CAD build for the part. Positions are in the model's coordinates, mm. Face numbers are marked on the shaded views. A direction names the side the tool comes from. Give positions to 0.01 mm unless a question says otherwise; leave off trailing zeros. Loops run counter-clockwise (first coordinate to the right, second up) from the corner with the lowest first, then second, coordinate; pieces in that order, holes last. Notation, with made-up numbers: M -12,28 L -8,28 A30 ccw -8,61 Z; hole C 43,87.25 d9. An arc over 180 degrees is marked long. One line per question, with ' | ' between items.
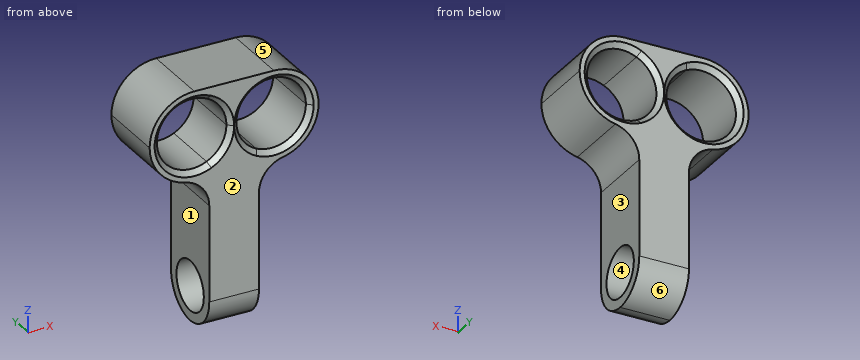
```python
from build123d import *

# Parameters (mm, degrees)
F0_W     = 5
F0_H     = 16
F1_DEPTH = 7
F3_D     = 5
F4_R     = 4.49999
F5_R     = 3.49999
F6_R     = 3
F7_SIZE  = 0.49999


# Not quite as in the source:
# - a fillet or chamfer is up to 0.001 mm smaller than in the source, because OpenCascade refuses the exact size


with BuildPart() as f1:
    # F0 (on Front) → F1 (new body)
    with BuildSketch(Plane.XZ):
        with BuildLine():
            Line((8.5, 12.5), (2.5, 12.5))
            Line((2.5, 12.5), (2.5, 11.1622776602))
            ThreePointArc((2.5, 11.1622776602), (5.8708286934, 10.9580398915), (7.5, 8))
            ThreePointArc((7.5, 8), (5.8708286934, 5.0419601085), (2.5, 4.8377223398))
            Line((2.5, 4.8377223398), (2.5, 3.5))
            Line((2.5, 3.5), (8.5, 3.5))
            Line((8.5, 3.5), (8.5, 12.5))
        make_face()
        with BuildLine():
            Line((-2.5, 11.1622776602), (-2.5, 12.5))
            Line((-2.5, 12.5), (-8.5, 12.5))
            Line((-8.5, 12.5), (-8.5, 3.5))
            Line((-8.5, 3.5), (-2.5, 3.5))
            Line((-2.5, 3.5), (-2.5, 4.8377223398))
            ThreePointArc((-2.5, 4.8377223398), (-7.5, 8), (-2.5, 11.1622776602))
        make_face()
        with BuildLine():
            Line((2.5, 11.1622776602), (2.5, 12.5))
            Line((2.5, 12.5), (-2.5, 12.5))
            Line((-2.5, 12.5), (-2.5, 11.1622776602))
            ThreePointArc((-2.5, 11.1622776602), (-1.0419601085, 9.8708286934), (-0.5, 8))
            ThreePointArc((-0.5, 8), (-1.0419601085, 6.1291713066), (-2.5, 4.8377223398))
            Line((-2.5, 4.8377223398), (-2.5, 3.5))
            Line((-2.5, 3.5), (2.5, 3.5))
            Line((2.5, 3.5), (2.5, 4.8377223398))
            ThreePointArc((2.5, 4.8377223398), (0.5, 8), (2.5, 11.1622776602))
        make_face()
        with Locations((0, -4.5)):
            Rectangle(F0_W, F0_H)
    extrude(amount=F1_DEPTH)

    # F3 (through all)
    with Locations(Plane.YZ.offset(2.5)):
        with Locations((-3.5, -9)):
            Hole(F3_D / 2)

    # F4 (radius 4.5 in the source; OpenCascade refuses exactly that, so slightly less here)
    f4_edges = [f1.edges().sort_by_distance(p)[0] for p in [
        (8.5, -3.5, 12.5),
        (-8.5, -3.5, 12.5),
        (8.5, -3.5, 3.5),
        (-8.5, -3.5, 3.5),
    ]]
    fillet(f4_edges, radius=F4_R)

    # F5 (radius 3.5 in the source; OpenCascade refuses exactly that, so slightly less here)
    f5_edges = [f1.edges().sort_by_distance(p)[0] for p in [
        (0, 0, -12.5),
        (0, -7, -12.5),
    ]]
    fillet(f5_edges, radius=F5_R)

    # F6
    f6_edges = [f1.edges().sort_by_distance(p)[0] for p in [
        (2.5, -3.5, 3.5),
        (-2.5, -3.5, 3.5),
    ]]
    fillet(f6_edges, radius=F6_R)

    # F7 (size 0.5 in the source; OpenCascade refuses exactly that, so slightly less here)
    f7_edges = [f1.edges().sort_by_distance(p)[0] for p in [
        (-7.5, -7, 8),
        (5.5, -7, 11.162278),
        (-7.5, 0, 8),
        (5.5, 0, 11.162278),
    ]]
    chamfer(f7_edges, length=F7_SIZE)


solid = f1.part
```
Item 1: Saw through at A-A on z = -10.5. Give the cut face in (x, y), and give its area (3 significant figures).
Conclusion:
outline: M -2.5,-6.66 L 2.5,-6.66 L 2.5,-5.5 L -2.5,-5.5 Z; M -2.5,-1.5 L 2.5,-1.5 L 2.5,-0.34 L -2.5,-0.34 Z | area: 11.6 mm²
Item 2: Saw through at B-B on x = 0.75. State how many separate pieces and enclosed holes the cut face has, and give its area (3 significant figures).
Conclusion:
separate pieces: 2 | enclosed holes: 1 | area: 131 mm²
Item 3: Drop flat-ended pins along their axis: P1, Ø1, axis at y = -1, z = 2, coming from the -X side; P2, Ø3.5, axis at y = -3.5, z = -3.5, coming from the +X side; P3, Ø1, axis at x = -1.5, y = -4.5, coming from the -Z side. Give the stop position or say it passes through.
Conclusion:
P1: x = -3.14 | P2: x = 2.5 | P3: z = -12.46
Item 4: 3-axis set-ups, long thin cutter, end or side, ignore diameter. For the marked faces 1, 2 and 3: which of +Z, -Z, +X, -X, +Y, -Y reach the whole face in a straight line?
Conclusion:
face 1: -Z, -X, +Y, -Y | face 2: +Z, -Z, +X, -X, -Y | face 3: -Z, +X, +Y, -Y
Item 5: Saw through at D-D on z = -6.75. Give the cut face in (x, y), and give its area (3 significant figures).
Conclusion:
outline: M -2.5,-7 L 2.5,-7 L 2.5,-4.59 L -2.5,-4.59 Z; M -2.5,-2.41 L 2.5,-2.41 L 2.5,0 L -2.5,0 Z | area: 24.1 mm²
Item 6: Mould opens along Z. For the marked faces 4, 5 and 6 say: pulls with the +Z half, pulls with the -Z half, needs draft (parallel to the pull), parting line crosses it, or undercut.
Conclusion:
face 4: undercut | face 5: pulls with the +Z half | face 6: pulls with the -Z half
Item 7: Drill centre lines: line 1 along X through (y, z) = (-5.75, 5.5); line 2 along X through (y, z) = (-1.5, 6.25); line 3 along Z through (x, y) = (-2, -5). Where is each one in solid material? Low to high. Write a range as [from, to].
Conclusion:
line 1: [-7.74, -6.45], [-1.55, 1.55], [6.45, 7.74] | line 2: [-8.15, -7.03], [-0.97, 0.97], [7.03, 8.15] | line 3: [-12.16, -11], [-7, 5.13], [10.87, 12.5]
